Design review of the part shown in the three views and the two pictorial views. Dimensions are in mm from the part's minimum x, y and z. Give positions to 0.01 mm unless a question says otherwise; leave off trailing zeros. Write each loop counter-clockwise with the first axis right and the second up, starting at its lowest first coordinate (ties: lowest second). Pieces come first, ordered by that corner, then holes.
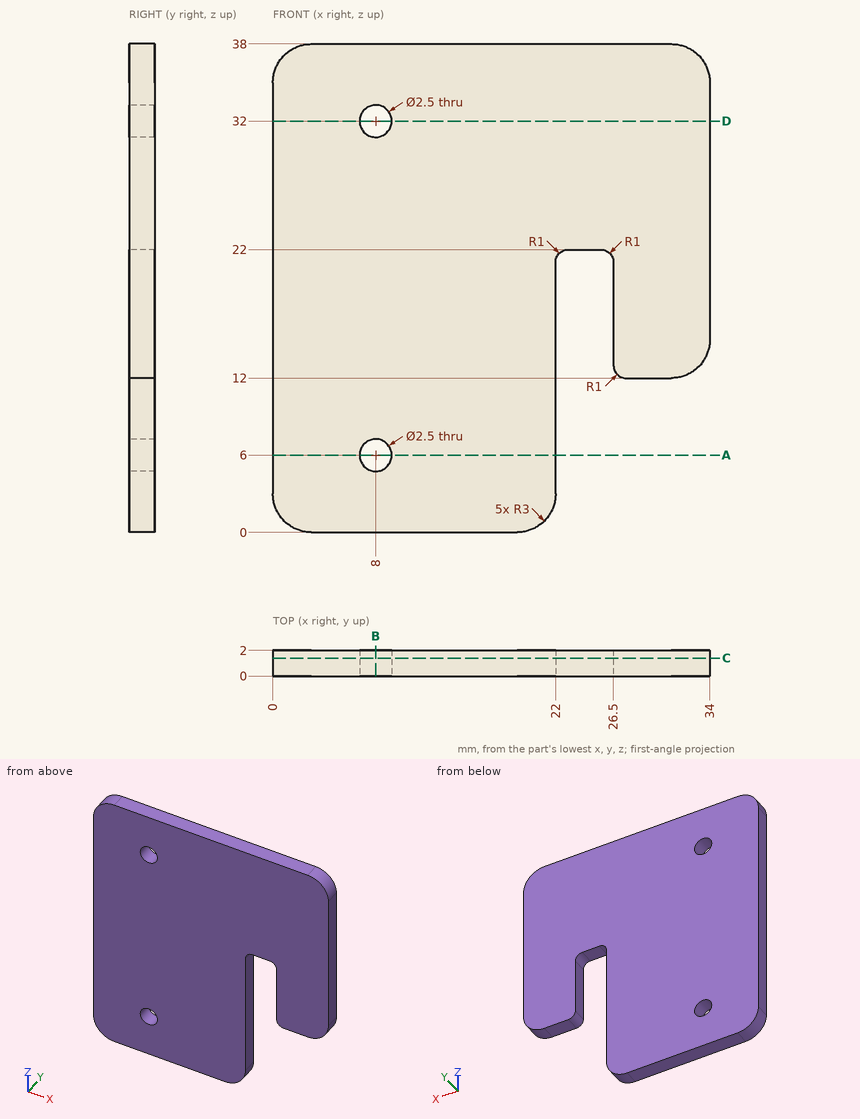
(1) Consider section D-D, the plane z = 32. Give the boundary of the cut face in (x, y), then the cut area to 3 significant figures.
Resolved:
outline: (0, 0) - (6.75, 0) - (6.75, 2) - (0, 2) - close; (9.25, 0) - (34, 0) - (34, 2) - (9.25, 2) - close
area: 63.0 mm2
(2) Clearance check with flat-ended pins moving along their axes: P1, Ø2, axis at x = 8, z = 6, coming from the +Y side; P2, Ø1, axis at x = 24, y = 0.5, coming from the -Z side. State where each tip first meets the part, or that it passes through.
Resolved:
P1: passes through
P2: stops at z = 22
(3) Consider section A-A, the plane z = 6. Give the boundary of the cut face in (x, y), then the cut area to 3 significant figures.
Resolved:
outline: (0, 0) - (6.75, 0) - (6.75, 2) - (0, 2) - close; (9.25, 0) - (22, 0) - (22, 2) - (9.25, 2) - close
area: 39.0 mm2
(4) Consider section B-B, the plane x = 8. Give the boundary of the cut face in (y, z), then the cut area to 3 significant figures.
Resolved:
outline: (0, 0) - (2, 0) - (2, 4.75) - (0, 4.75) - close; (0, 7.25) - (2, 7.25) - (2, 30.75) - (0, 30.75) - close; (0, 33.25) - (2, 33.25) - (2, 38) - (0, 38) - close
area: 66.0 mm2
(5) Consider section C-C, the plane y = 1.4. Give the boundary of the cut face in (x, z), then the cut area to 3 significant figures.
Resolved:
outline: (0, 3) arc R3 ccw to (3, 0) - (19, 0) arc R3 ccw to (22, 3) - (22, 21) arc R1 cw to (23, 22) - (25.5, 22) arc R1 cw to (26.5, 21) - (26.5, 13) arc R1 ccw to (27.5, 12) - (31, 12) arc R3 ccw to (34, 15) - (34, 35) arc R3 ccw to (31, 38) - (3, 38) arc R3 ccw to (0, 35) - close; hole circle Ø2.5 at (8, 6); hole circle Ø2.5 at (8, 32)
area: 1,080 mm2
(6) To check wall thickness, follow L1, parallel to Z at x = 8, y = 0.4; L2, parallel to X at y = 1.25, z = 6; L3, parallel to Z at x = 7.5, y = 1.05. State the ranges of each line that lie inside material, in increasing order.
Resolved:
L1: z = 0 to 4.75, 7.25 to 30.75, 33.25 to 38
L2: x = 0 to 6.75, 9.25 to 22
L3: z = 0 to 4.85, 7.15 to 30.85, 33.15 to 38
